The drawing under review shows one solid part. Ordinate dimensions are in mm from its lowest x, y, z. Round coordinates to 2 decimals unless told otherwise and drop trailing zeros. Write each loop counter-clockwise with the first axis right and the second up, starting at its lowest first coordinate (ties: lowest second). Pieces come first, ordered by that corner, then holes. Notation, with made-up numbers: M 86,72.25 L 127,72.25 A5 cw 127,76.25 Z; hole C 24,36 d8. An arc over 180 degrees is marked long. One line per item, written item: value. Start each with the question number.
1) Take a section at A-A, the plane y = 1.2. Write out the cut boundary in (x, z).
2) Take a section at D-D, the plane x = 9.5. Write out the cut boundary in (y, z).
3) Take a section at B-B, the plane z = 44. Write out the cut boundary in (x, y).
4) Wall thickness on probe 1 along X at (y, z) = (0.7, 44); probe 2 along X at (y, z) = (1.35, 5); probe 3 along Z at (x, y) = (9, 0.55): over which ranges is each line inside the solid? List them lowest first.
5) For P1, Ø4, axis at x = 4.5, z = 19, coming from the -Y side; P2, Ø1, axis at x = 2.5, y = 1, coming from the -Z side, all flat-tipped, find the tip position at first contact; note any pin that passes through.
6) Take a section at C-C, the plane x = 5.75. Write out the cut boundary in (y, z).
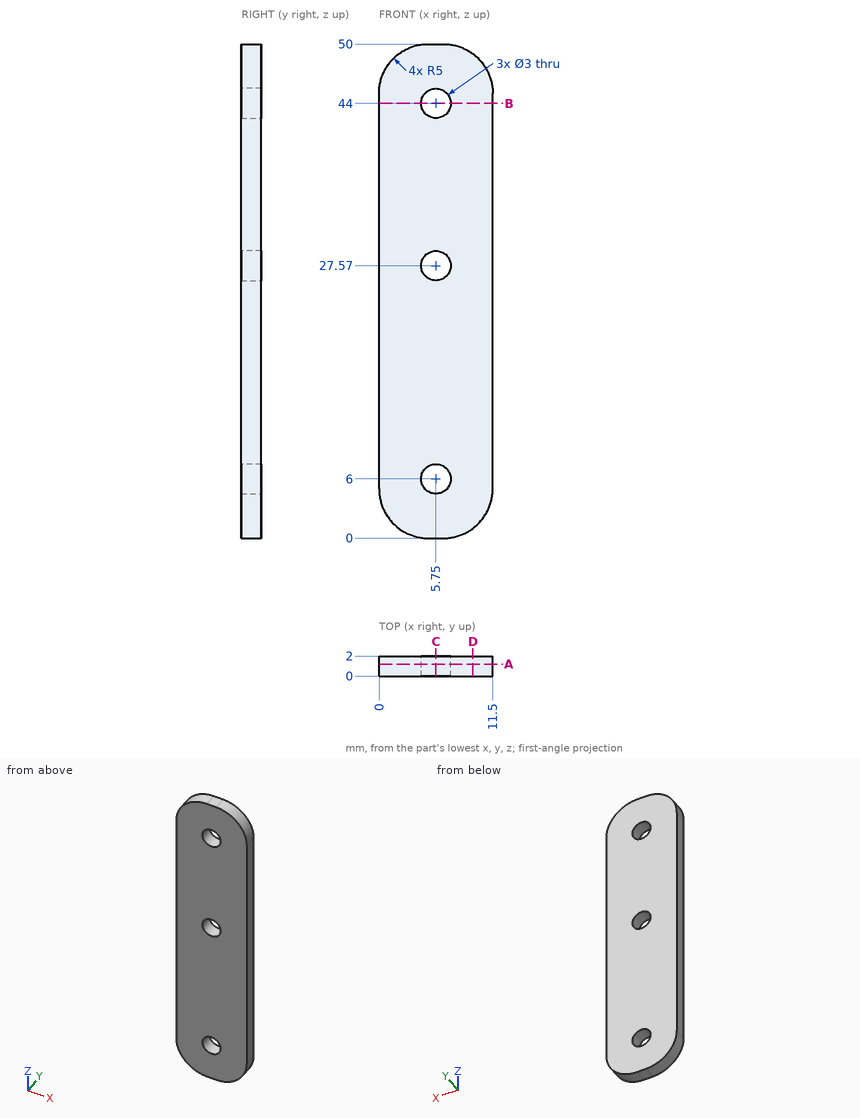
Checked values:
1. outline: M 0,5 A5 ccw 5,0 L 6.5,0 A5 ccw 11.5,5 L 11.5,45 A5 ccw 6.5,50 L 5,50 A5 ccw 0,45 Z; hole C 5.75,6 d3; hole C 5.75,27.57 d3; hole C 5.75,44 d3
2. outline: M 0,1 L 2,1 L 2,49 L 0,49 Z
3. outline: M 0,0 L 4.25,0 L 4.25,2 L 0,2 Z; M 7.25,0 L 11.5,0 L 11.5,2 L 7.25,2 Z
4. probe 1: x = 0 to 4.25, 7.25 to 11.5
4. probe 2: x = 0 to 4.63, 6.87 to 11.5
4. probe 3: z = 0.67 to 49.33
5. P1: stops at y = 0
5. P2: stops at z = 0.42
6. outline: M 0,0 L 2,0 L 2,4.5 L 0,4.5 Z; M 0,7.5 L 2,7.5 L 2,26.07 L 0,26.07 Z; M 0,29.07 L 2,29.07 L 2,42.5 L 0,42.5 Z; M 0,45.5 L 2,45.5 L 2,50 L 0,50 Z
